```python
from build123d import *

# Parameters (mm, degrees)
F1_DEPTH  = 2
F3_DEPTH  = 2
F5_DEPTH  = 2
F7_DEPTH  = 2
F9_DEPTH  = 2
F10_R     = 7.838323
F11_DEPTH = 2
F12_R     = 4.907322
F13_DEPTH = 25.4
F14_R     = 4.658547
F15_DEPTH = 5


with BuildPart() as f1:
    # F0 (on Top) → F1 (new body)
    with BuildSketch(Plane.XY):
        Polygon((25.346567, 25.346567), (0, 35.845459), (-25.346567, 25.346567), (-35.845459, 0), (-25.346567, -25.346567), (0, -35.845459), (25.346567, -25.346567), (35.845459, 0), align=None)
    extrude(amount=F1_DEPTH)

    # F2 (on face) → F3 (join)
    with BuildSketch(Plane.XY.offset(2)):
        Polygon((20.415665, 20.415665), (0, 28.87211), (-20.415665, 20.415665), (-28.87211, 0), (-20.415665, -20.415665), (0, -28.87211), (20.415665, -20.415665), (28.87211, 0), align=None)
    extrude(amount=F3_DEPTH)

    # F4 (on face) → F5 (join)
    with BuildSketch(Plane.XY.offset(4)):
        Polygon((14.96572, 14.96572), (0, 21.164725), (-14.96572, 14.96572), (-21.164725, 0), (-14.96572, -14.96572), (0, -21.164725), (14.96572, -14.96572), (21.164725, 0), align=None)
    extrude(amount=F5_DEPTH)

    # F6 (on face) → F7 (join)
    with BuildSketch(Plane.XY.offset(6)):
        Polygon((9.429269, 9.429269), (0, 13.335001), (-9.429269, 9.429269), (-13.335001, 0), (-9.429269, -9.429269), (0, -13.335001), (9.429269, -9.429269), (13.335001, 0), align=None)
    extrude(amount=F7_DEPTH)

    # F8 (on face) → F9 (join)
    with BuildSketch(Plane.XY.offset(8)):
        Polygon((5.27693, 5.27693), (0, 7.462706), (-5.27693, 5.27693), (-7.462706, 0), (-5.27693, -5.27693), (0, -7.462706), (5.27693, -5.27693), (7.462706, 0), align=None)
    extrude(amount=F9_DEPTH)

    # F10 (on Top) → F11 (join)
    with BuildSketch(Plane.XY):
        with Locations((0, 36.824174)):
            Circle(F10_R)
    extrude(amount=F11_DEPTH)

    # F12 (on face) → F13 (cut)
    with BuildSketch(Plane.XY.offset(2)):
        with Locations((0, 36.824174)):
            Circle(F12_R)
    extrude(amount=-F13_DEPTH, mode=Mode.SUBTRACT)

    # F14 (on face) → F15 (join)
    with BuildSketch(Plane.XY.offset(10)):
        Circle(F14_R)
    extrude(amount=F15_DEPTH)


solid = f1.part
```
Check sheet for the modelled part. Datum: model origin and axes. Units: mm. A direction names the side the tool comes from. Coordinates: 2 decimals unless noted, no trailing zeros. Order: outer loops, then holes, each group sorted by start corner. A loop starts at its lowest first (then second) coordinate and runs counter-clockwise, first axis right, second up. Notation, with made-up numbers: (-25.5, -8) -> (9.5, -8) arc R26 ccw to (9.5, 24) -> close; hole circle Ø10 at (15, -17). An arc over 180 degrees is marked (long way). Write each question's results on one line, items separated by ' | '. Start each with the question number.
1) Section check C-C (z = 13). Enter the section's corners in (x, y), and give its area (3 significant figures).
2) Draft check along Y on faces 1 (the face through (-11.41, -4.65, 6.99)), 2 (the face through (-1.064, 32.034, 1.014)), 3 (the face through (-18.02, 7.59, 4.99)), 4 (the face through (0.23, 44.66, 0.99)). Enter one of: pulls with the +Y half, pulls with the -Y half, needs draft (parallel to the pull), parting line crosses it, or undercut.
3) Section check A-A (x = -16). Enter the section's corners in (y, z), and give its area (3 significant figures).
4) Depth check by flat-ended pin: pin 1 (2 mm diameter, centred on x = 16, z = 4, fed in from +Y); pin 2 (5 mm diameter, centred on x = -28, y = -15.5, fed in from +Z); pin 3 (6 mm diameter, centred on y = -8.5, z = 8.5, fed in from +X); pin 4 (8 mm diameter, centred on x = 0, y = 36.82, fed in from +Z). Enter the tip coordinate at first touch or a pass-through.
5) Set-up check for faces 5 (the face through (-2.602, 6.385, 8.986)), 6 (the face through (-3.7, -2.83, 12.46)), 7 (the face through (4.65, -11.41, 6.99)), 8 (the face through (-7.59, -18.02, 4.99)): record each of +Z, -Z, +X, -X, +Y, -Y from which the full face is reachable in a straight line by a thin tool's end or side.
6) Material ranges on line 1 along Y through (x, z) = (0, 0.45); line 2 along Z through (x, y) = (9, 17.5); line 3 along Z through (x, y) = (29, -8.5), recorded low to high.
7) Section check B-B (y = 23). Enter the section's corners in (x, z), and give its area (3 significant figures).
Checked values:
1) outline: circle Ø9.32 at (0, 0) | area: 68.2 mm²
2) face 1: pulls with the -Y half | face 2: undercut | face 3: pulls with the +Y half | face 4: undercut
3) outline: (-29.22, 0) -> (29.22, 0) -> (29.22, 2) -> (22.24, 2) -> (22.24, 4) -> (12.47, 4) -> (12.47, 6) -> (-12.47, 6) -> (-12.47, 4) -> (-22.24, 4) -> (-22.24, 2) -> (-29.22, 2) -> close | area: 256 mm²
4) pin 1: y = 22.66 | pin 2: z = 2 | pin 3: x = 18.33 | pin 4: through
5) face 5: +Z, -X, +Y | face 6: +Z | face 7: +Z, +X, -Y | face 8: +Z, -X, -Y
6) line 1: -35.85 to 31.92, 41.73 to 44.66 | line 2: 0 to 4 | line 3: 0 to 2
7) outline: (-26.32, 0) -> (26.32, 0) -> (26.32, 2) -> (14.18, 2) -> (14.18, 4) -> (-14.18, 4) -> (-14.18, 2) -> (-26.32, 2) -> close | area: 162 mm²
